CAD build for the part. Positions are in the model's coordinates, mm. A direction names the side the tool comes from. Round coordinates to 2 decimals unless told otherwise and drop trailing zeros. Loops run counter-clockwise (first coordinate to the right, second up) from the corner with the lowest first, then second, coordinate; pieces in that order, holes last. Notation, with made-up numbers: (-13.5, 33.5) - (38.5, 33.5) arc R11 cw to (38.5, 47.5) - close; hole circle Ø8 at (75.25, -2). An arc over 180 degrees is marked (long way). Use one line per item in the form item = value.
from build123d import *

# Parameters (mm, degrees)
BOSS_EXTRUDE1_DEPTH             = 44.73702
BOSS_EXTRUDE1_DEPTH_BACK        = 44.73702
TAP_DRILL_FOR_1_4_20_TAP1_D     = 5.1054
TAP_DRILL_FOR_1_4_20_TAP1_DEPTH = 19.05
TAP_DRILL_FOR_1_4_20_TAP1_TIP   = 1.533816902
TAP_DRILL_FOR_1_4_20_TAP2_D     = 5.1054
TAP_DRILL_FOR_1_4_20_TAP2_DEPTH = 19.05
TAP_DRILL_FOR_1_4_20_TAP2_TIP   = 1.533816902


with BuildPart() as part:
    # Sketch3 → Boss-Extrude1 (new, two sides: drawn at the far end of the back side and taken through both)
    with BuildSketch(Plane.XY.offset(-BOSS_EXTRUDE1_DEPTH_BACK)):
        Polygon((0, 7.332348419), (-6.35, 3.666174209), (-6.35, -3.666174209), (0, -7.332348419), (6.35, -3.666174209), (6.35, 3.666174209), align=None)
    extrude(amount=BOSS_EXTRUDE1_DEPTH + BOSS_EXTRUDE1_DEPTH_BACK)

    # Tap Drill for 1/4-20 Tap1
    with Locations(Plane(origin=(0, 0, -44.73702), x_dir=(-1, 0, 0), z_dir=(0, 0, -1))):
        with Locations((0, 0)):
            Hole(TAP_DRILL_FOR_1_4_20_TAP1_D / 2, depth=TAP_DRILL_FOR_1_4_20_TAP1_DEPTH)
            with Locations((0, 0, -(TAP_DRILL_FOR_1_4_20_TAP1_DEPTH + TAP_DRILL_FOR_1_4_20_TAP1_TIP / 2))):  # 118° drill point
                Cone(0, TAP_DRILL_FOR_1_4_20_TAP1_D / 2, TAP_DRILL_FOR_1_4_20_TAP1_TIP, mode=Mode.SUBTRACT)

    # Tap Drill for 1/4-20 Tap2
    with Locations(Plane.XY.offset(44.73702)):
        with Locations((0, 0)):
            Hole(TAP_DRILL_FOR_1_4_20_TAP2_D / 2, depth=TAP_DRILL_FOR_1_4_20_TAP2_DEPTH)
            with Locations((0, 0, -(TAP_DRILL_FOR_1_4_20_TAP2_DEPTH + TAP_DRILL_FOR_1_4_20_TAP2_TIP / 2))):  # 118° drill point
                Cone(0, TAP_DRILL_FOR_1_4_20_TAP2_D / 2, TAP_DRILL_FOR_1_4_20_TAP2_TIP, mode=Mode.SUBTRACT)


solid = part.part
1) Tool access for faces 4 (the flat face through (0, -3, -44.737)), 5 (the cylindrical face through (2.435, 0.767, -35.079)): list every direction of +Z, -Z, +X, -X, +Y, -Y with a clear straight run to the whole face (end or side of a thin tool).
Report:
face_4 = -Z, +X, -X, +Y, -Y
face_5 = -Z
2) Slice it at B-B (z = -20). Write the cut outline in (x, y), plus the area to 3 significant figures.
Report:
outline = (-6.35, -3.67) - (0, -7.33) - (6.35, -3.67) - (6.35, 3.67) - (0, 7.33) - (-6.35, 3.67) - close
area = 140 mm^2
3) Flat gauge pin, fed straight in: pin 1 (2 mm diameter, centred on x = -3, z = 34.5, fed in from -Y). Where does the tip first touch, or does it go through?
Report:
pin_1 = -6.18
4) Slice it at D-D (y = -4.75). Write the cut outline in (x, z).
Report:
outline = (-4.47, -44.74) - (4.47, -44.74) - (4.47, 44.74) - (-4.47, 44.74) - close
5) Slice it at C-C (x = 4). Write the cut outline in (y, z).
Report:
outline = (-5.02, -44.74) - (5.02, -44.74) - (5.02, 44.74) - (-5.02, 44.74) - close
6) Drill centre lines: probe 1 along X at (y, z) = (0, 34.5); probe 2 along Y at (x, z) = (0, 32.5); probe 3 along Y at (x, z) = (-0.75, 35). Where is each one in solid material? Low to high.
Report:
probe_1 = -6.35 to -2.55, 2.55 to 6.35
probe_2 = -7.33 to -2.55, 2.55 to 7.33
probe_3 = -6.9 to -2.44, 2.44 to 6.9
7) Two-plate mould, pull along Y, no slides. Class faces 1 (the flat face through (3.131, -5.525, -0.626)), 2 (the flat face through (0, -3, 44.737)), 3 (the cylindrical face through (-2.435, 0.767, 35.079)): +Y half, -Y half, draft (parallel to the pull), parting line (faces both ways), or undercut.
Report:
face_1 = -Y half
face_2 = draft
face_3 = undercut
8) Slice it at A-A (z = 29). Write the cut outline in (x, y).
Report:
outline = (-6.35, -3.67) - (0, -7.33) - (6.35, -3.67) - (6.35, 3.67) - (0, 7.33) - (-6.35, 3.67) - close; hole circle Ø5.11 at (0, 0)
